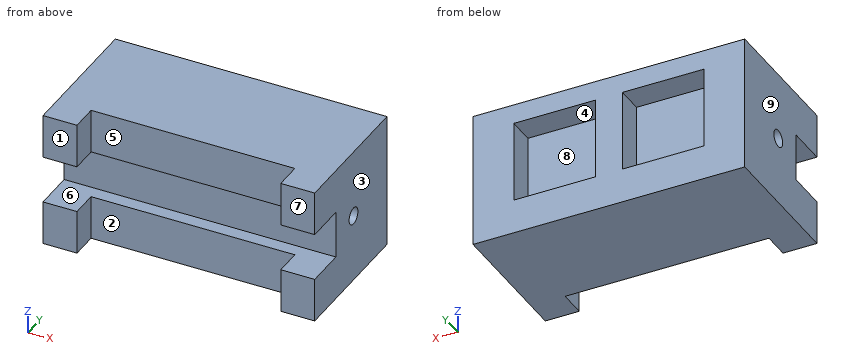
from build123d import *

# Parameters (mm, degrees)
EXTRUDE_1_DEPTH     = 40
SKETCH_2_R          = 2.5
SKETCH_2_W          = 14
SKETCH_2_H          = 12
CUT_EXTRUDE_1_DEPTH = 99.392072851
SKETCH_3_W          = 24
SKETCH_3_H          = 24
CUT_EXTRUDE_2_DEPTH = 8


with BuildPart() as part:
    # Эскиз1 → Бобышка-Вытянуть1 (new body)
    with BuildSketch(Plane.XY):
        Polygon((0, 0), (10, 0), (10, 8), (70, 8), (70, 0), (80, 0), (80, 41), (0, 41), align=None)
    extrude(amount=EXTRUDE_1_DEPTH)

    # Эскиз2 → Вырез-Вытянуть1 (cut, through all)
    with BuildSketch(Plane.ZY):
        with Locations((20, 22)):
            Circle(SKETCH_2_R)
        with Locations((20, 6)):
            Rectangle(SKETCH_2_W, SKETCH_2_H)
    extrude(amount=-CUT_EXTRUDE_1_DEPTH, mode=Mode.SUBTRACT)

    # Эскиз3 → Вырез-Вытянуть2 (cut)
    with BuildSketch(Plane(origin=(0, 41, 0), x_dir=(1, 0, 0), z_dir=(0, 1, 0))):
        with Locations((24, -22.220912541)):
            Rectangle(SKETCH_3_W, SKETCH_3_H)
        with Locations((56, -22.220912541)):
            Rectangle(SKETCH_3_W, SKETCH_3_H)
    extrude(amount=-CUT_EXTRUDE_2_DEPTH, mode=Mode.SUBTRACT)


solid = part.part
Check sheet for the modelled part. Datum: model origin and axes. Units: mm. Face numbers are marked on the shaded views. A direction names the side the tool comes from. Round coordinates to 2 decimals unless told otherwise and drop trailing zeros. Order: outer loops, then holes, each group sorted by start corner. A loop starts at its lowest first (then second) coordinate and runs counter-clockwise, first axis right, second up.
(1) Scan lines: probe 1 along X at (y, z) = (38, 28); probe 2 along Y at (x, z) = (63, 20); probe 3 along Y at (x, z) = (14.5, 14). Record each from-to range of solid material in increasing order.
(2) Draft check along X on the marked faces 1, 2, 3 and 4. Enter one of: pulls with the +X half, pulls with the -X half, needs draft (parallel to the pull), parting line crosses it, or undercut.
(3) Go/stop test with flat-tipped pins: P1, Ø4, axis at x = 32.5, z = 8, coming from the -Y side; P2, Ø5, axis at x = 32, z = 18, coming from the -Y side; P3, Ø12, axis at x = 55, z = 20, coming from the +Y side. Record where each tip stops, or that it passes through.
(4) Cross-section at A-A, the plane x = 42.5. Enter the section's corners in (y, z).
(5) Cross-section at B-B, the plane y = 22. Enter the section's corners in (x, z).
(6) Cross-section at C-C, the plane z = 20. Enter the section's corners in (x, y).
(7) Access from +Z, -Z, +X, -X, +Y, -Y to the whole of each face (thin tool, end or side, straight path). Record for the marked faces 5, 6, 7, 8 and 9.
(8) Cross-section at D-D, the plane y = 37.5. Enter the section's corners in (x, z).
Check sheet entries:
1. probe 1: x = 0 to 12, 36 to 44, 68 to 80
1. probe 2: y = 12 to 19.5, 24.5 to 33
1. probe 3: y = 12 to 33
2. face 1: needs draft
2. face 2: undercut
2. face 3: pulls with the +X half
2. face 4: undercut
3. P1: stops at y = 8
3. P2: stops at y = 12
3. P3: stops at y = 33
4. outline: (8, 0) - (41, 0) - (41, 40) - (8, 40) - (8, 27) - (12, 27) - (12, 13) - (8, 13) - close; hole circle Ø5 at (22, 20)
5. outline: (0, 0) - (80, 0) - (80, 17.5) - (0, 17.5) - close; (0, 22.5) - (80, 22.5) - (80, 40) - (0, 40) - close
6. outline: (0, 12) - (80, 12) - (80, 19.5) - (0, 19.5) - close; (0, 24.5) - (80, 24.5) - (80, 41) - (68, 41) - (68, 33) - (44, 33) - (44, 41) - (36, 41) - (36, 33) - (12, 33) - (12, 41) - (0, 41) - close
7. face 5: +Z, -Z, -Y
7. face 6: +X, -X, -Y
7. face 7: +Z, -Z, +X, -X, -Y
7. face 8: +Y
7. face 9: +Z, -Z, -X, +Y, -Y
8. outline: (0, 0) - (80, 0) - (80, 40) - (0, 40) - close; hole (12, 10.22) - (36, 10.22) - (36, 34.22) - (12, 34.22) - close; hole (44, 10.22) - (68, 10.22) - (68, 34.22) - (44, 34.22) - close
